```python
from build123d import *

# Parameters (mm, degrees)
ESQUISSE1_R        = 2.5
BOSS_EXTRU_1_DEPTH = 8
ESQUISSE2_R        = 2.75
BOSS_EXTRU_2_DEPTH = 0.7
ESQUISSE3_W        = 0.5
ESQUISSE3_H        = 0.5
BOSS_EXTRU_3_DEPTH = 10
CONG_1_R           = 2.5


with BuildPart() as part:
    # Esquisse1 → Boss.-Extru.1 (new body)
    with BuildSketch(Plane.XY):
        Circle(ESQUISSE1_R)
    extrude(amount=BOSS_EXTRU_1_DEPTH)

    # Esquisse2 → Boss.-Extru.2 (add)
    with BuildSketch(Plane.XY.offset(8)):
        Circle(ESQUISSE2_R)
    extrude(amount=BOSS_EXTRU_2_DEPTH)

    # Esquisse3 → Boss.-Extru.3 (add)
    with BuildSketch(Plane.XY.offset(8.7)):
        with Locations((-1.25, 0)):
            Rectangle(ESQUISSE3_W, ESQUISSE3_H)
        with Locations((1.25, 0)):
            Rectangle(ESQUISSE3_W, ESQUISSE3_H)
    extrude(amount=BOSS_EXTRU_3_DEPTH)

    # Congé1
    cong_1_edges = [part.edges().sort_by_distance(p)[0] for p in [
        (-2.5, 0, 0),
    ]]
    fillet(cong_1_edges, radius=CONG_1_R)


solid = part.part
```
For this review, take the finished solid that the model builds, in its own axes (mm). A direction names the side the tool comes from. Coordinates: 2 decimals unless noted, no trailing zeros. Write each loop counter-clockwise with the first axis right and the second up, starting at its lowest first coordinate (ties: lowest second). Pieces come first, ordered by that corner, then holes. Notation, with made-up numbers: (44.25, -35) -> (94.25, -35) arc R24 cw to (94.25, -2) -> close; hole circle Ø7 at (88, 25). An arc over 180 degrees is marked (long way). Put each result on its own line as item: value.
Q1. Take a section at B-B, the plane x = 0. State the section outline as (y, z) points.
From the geometry:
outline: (-2.75, 8) -> (-2.5, 8) -> (-2.5, 2.5) arc R2.5 ccw to (2.5, 2.5) -> (2.5, 8) -> (2.75, 8) -> (2.75, 8.7) -> (-2.75, 8.7) -> close
Q2. Take a section at A-A, the plane z = 9.5. State the section outline as (x, y) points, then the cut area to 3 significant figures.
From the geometry:
outline: (-1.5, -0.25) -> (-1, -0.25) -> (-1, 0.25) -> (-1.5, 0.25) -> close; (1, -0.25) -> (1.5, -0.25) -> (1.5, 0.25) -> (1, 0.25) -> close
area: 0.500 mm2
Q3. Wall thickness on L1, parallel to Y at x = -1.05, z = 17; L2, parallel to Z at x = -0.65, y = -0.75; L3, parallel to Z at x = -1.6, y = 1: over which ranges is each line inside the solid? List them lowest first.
From the geometry:
L1: y = -0.25 to 0.25
L2: z = 0.21 to 8.7
L3: z = 0.86 to 8.7
Q4. Take a section at C-C, the plane y = -1.65. State the section outline as (x, z) points, then the cut area to 3 significant figures.
From the geometry:
outline: (-2.2, 8) -> (-1.88, 8) -> (-1.88, 2.5) arc R1.88 ccw to (1.88, 2.5) -> (1.88, 8) -> (2.2, 8) -> (2.2, 8.7) -> (-2.2, 8.7) -> close
area: 29.3 mm2
Q5. Take a section at D-D, the plane z = 4.25. State the section outline as (x, y) points, then the cut area to 3 significant figures.
From the geometry:
outline: circle Ø5 at (0, 0)
area: 19.6 mm2
Q6. Tool access review of faces 1 (the cylindrical face through (-0.54, -2.44, 5.21)), 2 (the cylindrical face through (-0.596, -2.685, 8.345)): name each direction out of +Z, -Z, +X, -X, +Y, -Y from which nothing blocks a thin tool from reaching the whole face with its end or side.
From the geometry:
face 1: -Z
face 2: +Z, -Z
Q7. Clearance check with flat-ended pins moving along their axes: pin 1 Ø2 at (x, z) = (0.5, 12) entering from -Y; pin 2 Ø3 at (x, y) = (0, -0.5) entering from +Z; pin 3 Ø1 at (y, z) = (1.5, 9) entering from +X; pin 4 Ø1.6 at (x, y) = (-0.5, -1) entering from +Z. State where each tip first meets the part, or that it passes through.
From the geometry:
pin 1: stops at y = -0.25
pin 2: stops at z = 18.7
pin 3: stops at x = 2.52
pin 4: stops at z = 8.7
